Verification items for the finished model (mm, model axes). Give positions to 0.01 mm unless a question says otherwise; leave off trailing zeros. Write each loop counter-clockwise with the first axis right and the second up, starting at its lowest first coordinate (ties: lowest second). Pieces come first, ordered by that corner, then holes. Notation, with made-up numbers: M 10,-13 L 54,-13 A18 ccw 54,10 Z; hole C -3,40 d10. An arc over 180 degrees is marked long. Write item = value, one per line.
from build123d import *

# Parameters (mm, degrees)
F1_DEPTH      = 25
F4_ANGLE_BACK = 15
F4_ANGLE      = 30
F6_DEPTH      = 4.2


with BuildPart() as f1:
    # F0 (on Front) → F1 (new body)
    with BuildSketch(Plane.XZ):
        with BuildLine():
            ThreePointArc((26.3431364877, 8.5707053028), (25.1879544986, 13.2060879092), (21.0133194591, 15.5285089783))
            ThreePointArc((21.0133194591, 15.5285089783), (-0.0894086287, 17.0460813995), (-21.2428583947, 17.4457334904))
            ThreePointArc((-21.2428583947, 17.4457334904), (-27.0252643869, 15.3277245971), (-30.1521339791, 10.0225509634))
            ThreePointArc((-30.1521339791, 10.0225509634), (-30.737948683, -1.5598670025), (-28.1338702514, -12.8609448416))
            ThreePointArc((-28.1338702514, -12.8609448416), (-24.6579753008, -18.0246958087), (-19.2665178824, -21.1357015406))
            ThreePointArc((-19.2665178824, -21.1357015406), (-5.5690318774, -23.5254263951), (8.2977543738, -22.503591381))
            ThreePointArc((8.2977543738, -22.503591381), (13.1377213939, -20.4559972218), (16.7715565718, -16.6595298512))
            ThreePointArc((16.7715565718, -16.6595298512), (22.8064529235, -4.5182850542), (26.3431364877, 8.5707053028))
        make_face()
    extrude(amount=-F1_DEPTH)


with BuildPart() as f4:
    # F3 (on offset) → F4 (revolve)
    with BuildSketch(Plane.XY.offset(22), mode=Mode.PRIVATE) as f4_sk:
        with BuildLine():
            Line((-282, -293), (318, -293))
            ThreePointArc((318, -293), (18, 7), (-282, -293))
        make_face()
    revolve(f4_sk.sketch.rotate(Axis((18, -293, 22), (1, 0, 0)), -F4_ANGLE_BACK), axis=Axis((18, -293, 22), (1, 0, 0)), revolution_arc=F4_ANGLE)


with BuildPart() as f1_1:
    add(f1.part)

    # F5: intersect F4
    add(f4.part, mode=Mode.INTERSECT)

    # F6 (add): a face of the model
    f6_faces = [f1_1.faces().sort_by_distance(p)[0] for p in [
        (-3.417701973, 0, -1.7255808381),
    ]]
    extrude(f6_faces, amount=F6_DEPTH)


solid = f1_1.part
1) Cross-section at D-D on y = 2.25. Record the boundary of the cut face in (x, z) (1 decimal), plus the area to 3 significant figures.
From the geometry:
outline = M -30.9,1.1 A53.2 ccw -10.2,-23.1 A56.6 ccw 8.3,-22.5 A13 ccw 16.8,-16.7 A68.8 ccw 26.3,8.6 A6 ccw 21,15.5 A400 ccw -21.2,17.4 A9.1 ccw -30.2,10 A42 ccw Z
area = 1,880 mm^2
2) Material ranges on probe 1 along Y at (x, z) = (-12.5, 15.5); probe 2 along Y at (x, z) = (-22, -18); probe 3 along Z at (x, y) = (5, 2.5), recorded low to high. Write a range as from..to.
From the geometry:
probe_1 = -4.2..5.37
probe_2 = -4.2..1.62
probe_3 = -23.06..16.78
3) Cross-section at C-C on x = 6. Record the boundary of the cut face in (y, z), plus the area to 3 significant figures.
From the geometry:
outline = M -4.2,-22.91 L 3.38,-22.91 A299.76 ccw 6.71,16.72 L -4.2,16.72 Z
area = 384 mm^2
4) Cross-section at A-A on y = -3. Record the boundary of the cut face in (x, z) (1 decimal).
From the geometry:
outline = M -30.2,10 A42 ccw -28.1,-12.9 A13.8 ccw -19.3,-21.1 A56.6 ccw 8.3,-22.5 A13 ccw 16.8,-16.7 A68.8 ccw 26.3,8.6 A6 ccw 21,15.5 A400 ccw -21.2,17.4 A9.1 ccw Z
5) Depth check by flat-ended pin: P1, Ø4, axis at y = 3, z = -3.5, coming from the -X side; P2, Ø6, axis at x = 20, y = -2, coming from the +Z side; P3, Ø5, axis at x = -13.5, y = 2, coming from the +Z side; P4, Ø5, axis at y = -2.5, z = 8.5, coming from the +X side. Enter the tip coordinate at first touch or a pass-through.
From the geometry:
P1 = -30.72
P2 = 15.9
P3 = 17.45
P4 = 26.42
6) Cross-section at B-B on z = -2. Record the boundary of the cut face in (x, y).
From the geometry:
outline = M -30.7,-4.2 L 23.71,-4.2 L 23.71,5.98 A299.04 ccw -30.7,2.05 Z
